```python
from build123d import *

# Parameters (mm, degrees)
F0_W     = 140
F0_H     = 140
F1_DEPTH = 2
F2_R     = 2.5
F3_DEPTH = 25
F4_R     = 10


with BuildPart() as f1:
    # F0 (on Front) → F1 (new body)
    with BuildSketch(Plane.XZ):
        Rectangle(F0_W, F0_H)
    extrude(amount=F1_DEPTH)

    # F2 (on face) → F3 (cut)
    with BuildSketch(Plane.XZ.offset(2)):
        with Locations((-50, 50)):
            Circle(F2_R)
        with Locations((50, 50)):
            Circle(F2_R)
        with Locations((-50, -50)):
            Circle(F2_R)
        with Locations((50, -50)):
            Circle(F2_R)
    extrude(amount=-F3_DEPTH, mode=Mode.SUBTRACT)

    # F4
    f4_edges = [f1.edges().sort_by_distance(p)[0] for p in [
        (70, -1, 70),
        (70, -1, -70),
        (-70, -1, 70),
        (-70, -1, -70),
    ]]
    fillet(f4_edges, radius=F4_R)


solid = f1.part
```
The listing builds one solid part. Answer for the finished solid, in the listing's coordinates (mm). Coordinates: 2 decimals unless noted, no trailing zeros. Loops run counter-clockwise (first coordinate to the right, second up) from the corner with the lowest first, then second, coordinate; pieces in that order, holes last. Notation, with made-up numbers: (-18.5, 75.5) - (25.5, 75.5) arc R13 ccw to (25.5, 100.5) - close; hole circle Ø11 at (86.5, 16). An arc over 180 degrees is marked (long way). Use a Markdown table: item, result. Add a question column.
1) Given pin 1 (8 mm diameter, centred on x = -50, z = -50, fed in from -Y); pin 2 (3 mm diameter, centred on x = 50, z = -50, fed in from -Y), each flat-ended and moving along its own axis, determine where each tip first touches the part or whether it passes through.
2) The part is cut by section B-B, the plane z = 50. Give the vertices of the cut face in (x, y).
3) Find the intervals of material crossed by line 1 (Z direction, x = -50, y = -0.45); line 2 (X direction, y = -0.25, z = 49); line 3 (X direction, y = -0.1, z = -61), in increasing order.
4) The part is cut by section A-A, the plane x = 50. Give the vertices of the cut face in (y, z).
5) The mould has two halves that part along Z. Classify faces 1 (the flat face through (-1, 0, 1)), 2 (the cylindrical face through (66.99, -1.01, 67.15)), 3 (the cylindrical face through (52.31, -1.01, 49.04)): released by +Z, released by -Z, zero draft, split by the parting line, or undercut.
Here are the results:
| question | item | result |
|---|---|---|
| 1 | pin 1 | stops at y = -2 |
| 1 | pin 2 | passes through |
| 2 | outline | (-70, -2) - (-52.5, -2) - (-52.5, 0) - (-70, 0) - close; (-47.5, -2) - (47.5, -2) - (47.5, 0) - (-47.5, 0) - close; (52.5, -2) - (70, -2) - (70, 0) - (52.5, 0) - close |
| 3 | line 1 | z = -70 to -52.5, -47.5 to 47.5, 52.5 to 70 |
| 3 | line 2 | x = -70 to -52.29, -47.71 to 47.71, 52.29 to 70 |
| 3 | line 3 | x = -69.95 to 69.95 |
| 4 | outline | (-2, -70) - (0, -70) - (0, -52.5) - (-2, -52.5) - close; (-2, -47.5) - (0, -47.5) - (0, 47.5) - (-2, 47.5) - close; (-2, 52.5) - (0, 52.5) - (0, 70) - (-2, 70) - close |
| 5 | face 1 | zero draft |
| 5 | face 2 | released by +Z |
| 5 | face 3 | undercut |
